Input: part model. Units: mm. Frame: model coordinates. A direction names the side the tool comes from. Round coordinates to 2 decimals unless told otherwise and drop trailing zeros. Loops run counter-clockwise (first coordinate to the right, second up) from the corner with the lowest first, then second, coordinate; pieces in that order, holes last. Notation, with made-up numbers: M 37,62 L 69,62 A18 ccw 69,67 Z; hole C 56.25,46 d6. An arc over 180 degrees is marked long. Use one line per item in the form item = value. Start each with the question number.
Q1. Section query D-D, the plane z = -1.05. Output: boundary loops of the cut face in (x, y), and give its area (3 significant figures).
Q2. Section query C-C, the plane y = -5.25. Output: boundary loops of the cut face in (x, z).
Q3. Section query A-A, the plane x = 0. Output: boundary loops of the cut face in (y, z).
Q4. Ray query, line 1 along Y through (x, z) = (-0.55, -0.25); line 2 along X through (y, z) = (5.25, -0.1); line 3 along Z through (x, y) = (0.8, 6.25). Return the intervals inside material, ascending.
Q5. Access query for faces 1 (the flat face through (1, 0, 0)), 2 (the flat face through (0, 8, 1.05)), 3 (the flat face through (0, 10.7, 0)). Directions: +Z, -Z, +X, -X, +Y, -Y. A direction counts if a zero-diameter tool reaches every point of the face in a straight line with its end or side. Return the directions, or none.
Q6. Section query B-B, the plane z = 0. Output: boundary loops of the cut face in (x, y).
```python
from build123d import *

# Parameters (mm, degrees)
CROQUIS1_R              = 1.45
SALIENTE_EXTRUIR1_DEPTH = 10.7
CORTAR_EXTRUIR1_DEPTH   = 6
CROQUIS3_R              = 0.5
SALIENTE_EXTRUIR2_DEPTH = 6.4


with BuildPart() as part:
    # Croquis1 → Saliente-Extruir1 (new body)
    with BuildSketch(Plane(origin=(0, 0, 0), x_dir=(1, 0, 0), z_dir=(0, 1, 0))):
        Circle(CROQUIS1_R)
    extrude(amount=SALIENTE_EXTRUIR1_DEPTH)

    # Croquis2 → Cortar-Extruir1 (cut)
    with BuildSketch(Plane(origin=(0, 10.7, 0), x_dir=(1, 0, 0), z_dir=(0, 1, 0))):
        with BuildLine():
            Line((-1, -1.05), (1, -1.05))
            ThreePointArc((1, -1.05), (0, -1.45), (-1, -1.05))
        make_face()
    extrude(amount=-CORTAR_EXTRUIR1_DEPTH, mode=Mode.SUBTRACT)

    # Croquis3 → Saliente-Extruir2 (add)
    with BuildSketch(Plane.XZ):
        Circle(CROQUIS3_R)
    extrude(amount=SALIENTE_EXTRUIR2_DEPTH)


solid = part.part
```
Results found:
q1.outline = M -1,0 L 1,0 L 1,10.7 L -1,10.7 Z
q1.area = 21.4 mm²
q2.outline = C 0,0 d1
q3.outline = M -6.4,-0.5 L 0,-0.5 L 0,-1.45 L 10.7,-1.45 L 10.7,1.05 L 4.7,1.05 L 4.7,1.45 L 0,1.45 L 0,0.5 L -6.4,0.5 Z
q4.line_1 = 0 to 10.7
q4.line_2 = -1.45 to 1.45
q4.line_3 = -1.21 to 1.05
q5.face_1 = -Y
q5.face_2 = +Z, +X, -X, +Y
q5.face_3 = +Z, -Z, +X, -X, +Y
q6.outline = M -1.45,0 L -0.5,0 L -0.5,-6.4 L 0.5,-6.4 L 0.5,0 L 1.45,0 L 1.45,10.7 L -1.45,10.7 Z
